For this review, take the finished solid that the model builds, in its own axes (mm). A direction names the side the tool comes from. Round coordinates to 2 decimals unless told otherwise and drop trailing zeros. Loops run counter-clockwise (first coordinate to the right, second up) from the corner with the lowest first, then second, coordinate; pieces in that order, holes last.
```python
from build123d import *

# Parameters (mm, degrees)
FSAE_CHASSIS_MCMASTER_4130_1IN_X_065IN_DEPTH = 40
CUT_EXTRUDE1_DEPTH                           = 50.055580722
CUT_EXTRUDE1_DEPTH_BACK                      = 50.055580722
SKETCH3_R                                    = 6.4
CUT_EXTRUDE2_DEPTH                           = 50.055580722
CUT_EXTRUDE2_DEPTH_BACK                      = 50.055580722
FILLET1_R                                    = 2


with BuildPart() as part:
    # Sketch2 → Fsae chassis MCMASTER 4130 1IN X .065IN SQUARE STOCK(1) (new body)
    with BuildSketch(Plane.ZX):
        with BuildLine():
            Line((11.049, 12.7), (-11.049, 12.7))
            ThreePointArc((-11.049, 12.7), (-12.216433296, 12.216433296), (-12.7, 11.049))
            Line((-12.7, 11.049), (-12.7, -11.049))
            ThreePointArc((-12.7, -11.049), (-12.216433296, -12.216433296), (-11.049, -12.7))
            Line((-11.049, -12.7), (11.049, -12.7))
            ThreePointArc((11.049, -12.7), (12.216433296, -12.216433296), (12.7, -11.049))
            Line((12.7, -11.049), (12.7, 11.049))
            ThreePointArc((12.7, 11.049), (12.216433296, 12.216433296), (11.049, 12.7))
        make_face()
        with BuildLine():
            Line((-9.398, 11.049), (9.398, 11.049))
            ThreePointArc((9.398, 11.049), (10.565433296, 10.565433296), (11.049, 9.398))
            Line((11.049, 9.398), (11.049, -9.398))
            ThreePointArc((11.049, -9.398), (10.565433296, -10.565433296), (9.398, -11.049))
            Line((9.398, -11.049), (-9.398, -11.049))
            ThreePointArc((-9.398, -11.049), (-10.565433296, -10.565433296), (-11.049, -9.398))
            Line((-11.049, -9.398), (-11.049, 9.398))
            ThreePointArc((-11.049, 9.398), (-10.565433296, 10.565433296), (-9.398, 11.049))
        make_face(mode=Mode.SUBTRACT)
    extrude(amount=FSAE_CHASSIS_MCMASTER_4130_1IN_X_065IN_DEPTH)

    # Sketch3 → Cut-Extrude1 (cut, two sides: drawn at the far end of the back side and taken through both)
    with BuildSketch(Plane.XY.offset(12.7).offset(-CUT_EXTRUDE1_DEPTH_BACK)):
        with Locations((0, 12)):
            Circle(SKETCH3_R)
    extrude(amount=CUT_EXTRUDE1_DEPTH + CUT_EXTRUDE1_DEPTH_BACK, mode=Mode.SUBTRACT)

    # Sketch4 → Cut-Extrude2 (cut, two sides: drawn at the far end of the back side and taken through both)
    with BuildSketch(Plane(origin=(12.7, 0, 0), x_dir=(0, 0, -1), z_dir=(1, 0, 0)).offset(-CUT_EXTRUDE2_DEPTH_BACK)):
        with BuildLine():
            Line((-7.5, 0), (7.5, 0))
            Line((7.5, 0), (5.956316627, 12.722697892))
            ThreePointArc((5.956316627, 12.722697892), (0, 18), (-5.956316627, 12.722697892))
            Line((-5.956316627, 12.722697892), (-7.5, 0))
        make_face()
    extrude(amount=CUT_EXTRUDE2_DEPTH + CUT_EXTRUDE2_DEPTH_BACK, mode=Mode.SUBTRACT)

    # Fillet1
    fillet1_edges = [part.edges().sort_by_distance(p)[0] for p in [
        (11.8745, 0, 7.5),
        (11.8745, 0, -7.5),
        (-11.8745, 0, -7.5),
        (-11.8745, 0, 7.5),
    ]]
    fillet(fillet1_edges, radius=FILLET1_R)


solid = part.part
```
(1) Add section D-D (x = 0). Give the boundary of the cut face in (y, z), plus the area to 3 significant figures.
(2) The part is to be moulded in two halves that separate along Y. For faces 4 (the cylindrical face through (-1.387, 5.752, 11.863)), 5 (the flat face through (-11.049, 24, 0)), 6 (the flat face through (-11.89, 7.16, -6.63)), 7 (the cylindrical face through (-1.387, 5.752, -11.886)), say which applies: pulls with the +Y half, pulls with the -Y half, needs draft (parallel to the pull), parting line crosses it, or undercut.
(3) Add section B-B (y = 36). Give the boundary of the cut face in (x, z).
(4) For L1, parallel to Y at x = 0, z = -11.7; L2, parallel to Z at x = 3.5, y = 23, list the stretches that pass through material, from the lowest coordinate up.
(5) Add section C-C (z = -8.75). Give the boundary of the cut face in (x, y).
(6) Insertion check: pin 1 Ø11.5 at (x, y) = (0, 12) entering from +Z. The pin has a flat end and moves straight along its axis. Give the tip position at first contact, or say it passes through.
(7) Add section A-A (x = 8.75). Give the boundary of the cut face in (y, z), plus the area to 3 significant figures.
(8) For faces 1 (the cylindrical face through (11.89, 0.49, 7.96)), 2 (the flat face through (0, 20, -11.049)), 3 (the flat face through (0, 0, 12)), list the 3-axis set-ups (+Z, -Z, +X, -X, +Y, -Y) from which the entire face can be reached by the end or side of a thin tool; tool diameter is ignored.
Outcome:
1. outline: (0, -12.7) - (5.6, -12.7) - (5.6, -11.05) - (0, -11.05) - close; (0, 11.05) - (5.6, 11.05) - (5.6, 12.7) - (0, 12.7) - close; (18.4, -12.7) - (40, -12.7) - (40, -11.05) - (18.4, -11.05) - close; (18.4, 11.05) - (40, 11.05) - (40, 12.7) - (18.4, 12.7) - close
1. area: 89.8 mm2
2. face 4: undercut
2. face 5: needs draft
2. face 6: pulls with the -Y half
2. face 7: undercut
3. outline: (-12.7, -11.05) arc R1.65 ccw to (-11.05, -12.7) - (11.05, -12.7) arc R1.65 ccw to (12.7, -11.05) - (12.7, 11.05) arc R1.65 ccw to (11.05, 12.7) - (-11.05, 12.7) arc R1.65 ccw to (-12.7, 11.05) - close; hole (-11.05, -9.4) arc R1.65 ccw to (-9.4, -11.05) - (9.4, -11.05) arc R1.65 ccw to (11.05, -9.4) - (11.05, 9.4) arc R1.65 ccw to (9.4, 11.05) - (-9.4, 11.05) arc R1.65 ccw to (-11.05, 9.4) - close
4. L1: y = 0 to 5.6, 18.4 to 40
4. L2: z = -12.7 to -11.05, 11.05 to 12.7
5. outline: (-12.7, 0.07) - (-11.05, 0.07) - (-11.05, 40) - (-12.7, 40) - close; (11.05, 0.07) - (12.7, 0.07) - (12.7, 40) - (11.05, 40) - close
6. pin 1: passes through
7. outline: (0, -12.7) - (40, -12.7) - (40, -11.05) - (0, -11.05) - close; (0, 11.05) - (40, 11.05) - (40, 12.7) - (0, 12.7) - close
7. area: 132 mm2
8. face 1: +X, -X, -Y
8. face 2: +Y, -Y
8. face 3: +Z, -Z, +X, -X, -Y
